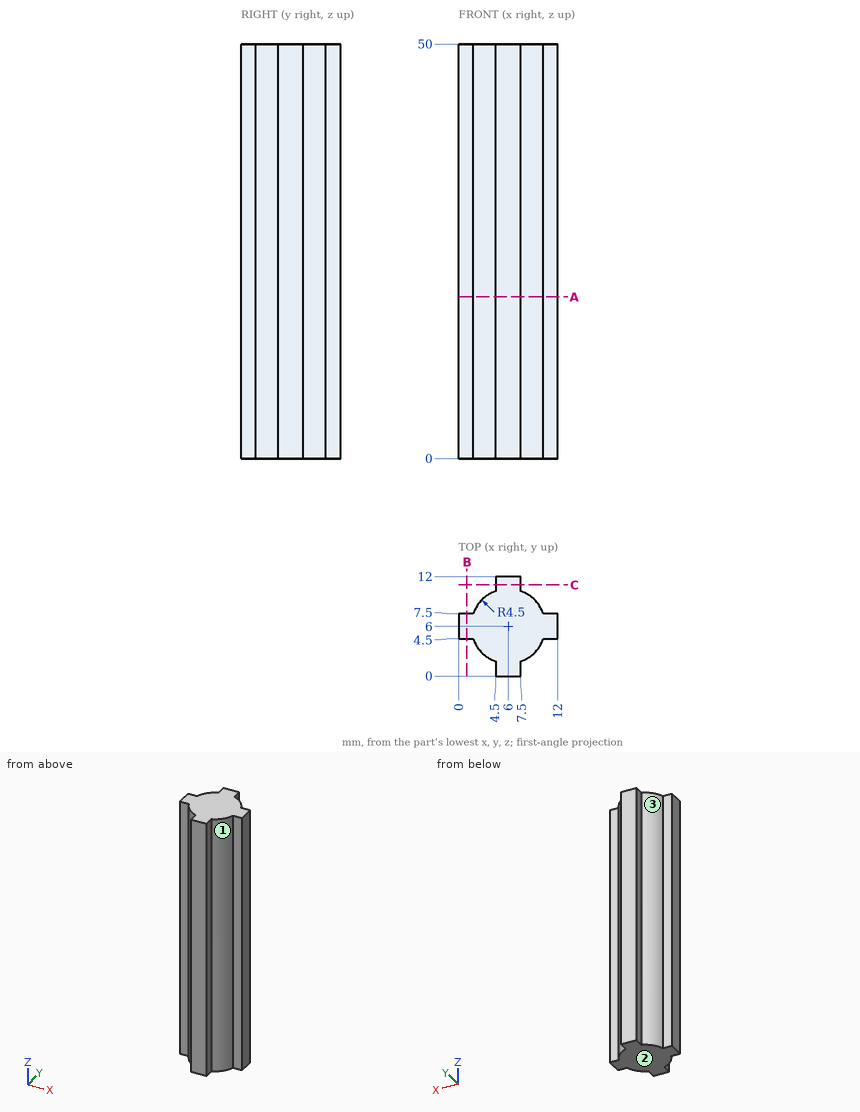
Here's the drawing with two shaded views (mm, measured from the low corner). I have some questions. Coordinates: 2 decimals unless noted, no trailing zeros. Write each loop counter-clockwise with the first axis right and the second up, starting at its lowest first coordinate (ties: lowest second). Pieces come first, ordered by that corner, then holes.
Item 1: I want a section at A-A on z = 19.5. Write out the boundary of the cut face in (x, y).
Item 2: If we mould it in two halves opening along X, with no side actions, what happens to the marked faces 1, 2 and 3? For each: +X half, -X half, draft (parallel to the pull), parting line (faces both ways), or undercut.
Item 3: Will these pins go through, and if not, where does the flat tip stop? pin 1 (0.5 mm diameter, centred on x = 0.5, z = 24, fed in from +Y); pin 2 (0.5 mm diameter, centred on y = 1, z = 31.5, fed in from +X); pin 3 (1 mm diameter, centred on x = 8.5, z = 12.5, fed in from +Y).
Item 4: I want a section at B-B on x = 1. Write out the boundary of the cut face in (y, z).
Item 5: If I drill on line 1 (X direction, y = 1, z = 45); line 2 (X direction, y = 8.5, z = 20), over which ranges is the centre line in solid material (lowest first)?
Findings below:
1. outline: (0, 4.5) - (1.76, 4.5) arc R4.5 ccw to (4.5, 1.76) - (4.5, 0) - (7.5, 0) - (7.5, 1.76) arc R4.5 ccw to (10.24, 4.5) - (12, 4.5) - (12, 7.5) - (10.24, 7.5) arc R4.5 ccw to (7.5, 10.24) - (7.5, 12) - (4.5, 12) - (4.5, 10.24) arc R4.5 ccw to (1.76, 7.5) - (0, 7.5) - close
2. face 1: +X half
2. face 2: draft
2. face 3: -X half
3. pin 1: stops at y = 7.5
3. pin 2: stops at x = 7.5
3. pin 3: stops at y = 10.03
4. outline: (4.5, 0) - (7.5, 0) - (7.5, 50) - (4.5, 50) - close
5. line 1: x = 4.5 to 7.5
5. line 2: x = 2.26 to 9.74
